```python
from build123d import *

# Parameters (mm, degrees)
SKETCH_1_R          = 1.5
EXTRUDE_2_DEPTH     = 5
CUT_EXTRUDE_2_DEPTH = 1
SKETCH_4_W          = 20
SKETCH_4_H          = 40
EXTRUDE_3_DEPTH     = 3


with BuildPart() as part:
    # 草图1 → 凸台-拉伸2 (new body)
    with BuildSketch(Plane(origin=(0, 0, 0), x_dir=(0, 0, -1), z_dir=(1, 0, 0))):
        with BuildLine():
            Line((-15, 0), (15, 0))
            Line((15, 0), (15, 130))
            ThreePointArc((15, 130), (16.060667235, 133.763397528), (17.833287426, 137.248507798))
            Line((17.833287426, 137.248507798), (34.277601095, 169.80605943))
            ThreePointArc((34.277601095, 169.80605943), (22.969406924, 178.256928012), (10.37531975, 171.878730504))
            Line((10.37531975, 171.878730504), (-12.166712574, 127.248507798))
            ThreePointArc((-12.166712574, 127.248507798), (-13.939332765, 123.763397528), (-15, 120))
            Line((-15, 120), (-15, 0))
        make_face()
        with Locations((0, 23.934052351)):
            Circle(SKETCH_1_R, mode=Mode.SUBTRACT)
        with Locations((0, 47.934052351)):
            Circle(SKETCH_1_R, mode=Mode.SUBTRACT)
        with Locations((0, 71.934052351)):
            Circle(SKETCH_1_R, mode=Mode.SUBTRACT)
        with Locations((0, 95.934052351)):
            Circle(SKETCH_1_R, mode=Mode.SUBTRACT)
        with Locations((10.541707006, 142.602806473)):
            Circle(SKETCH_1_R, mode=Mode.SUBTRACT)
        with Locations((0, 119.934052351)):
            Circle(SKETCH_1_R, mode=Mode.SUBTRACT)
        with Locations((21.812723168, 164.917917825)):
            Circle(SKETCH_1_R, mode=Mode.SUBTRACT)
        with Locations((11.964645637, 166.654399602)):
            Circle(SKETCH_1_R, mode=Mode.SUBTRACT)
        with Locations((11.964645637, 163.181436049)):
            Circle(SKETCH_1_R, mode=Mode.SUBTRACT)
        with Locations((13.15246913, 159.917917825)):
            Circle(SKETCH_1_R, mode=Mode.SUBTRACT)
        with Locations((15.384847071, 157.257473394)):
            Circle(SKETCH_1_R, mode=Mode.SUBTRACT)
        with Locations((21.812723168, 154.917917825)):
            Circle(SKETCH_1_R, mode=Mode.SUBTRACT)
        with Locations((18.392521734, 155.520991617)):
            Circle(SKETCH_1_R, mode=Mode.SUBTRACT)
        with Locations((13.15246913, 169.917917825)):
            Circle(SKETCH_1_R, mode=Mode.SUBTRACT)
        with Locations((15.384847071, 172.578362256)):
            Circle(SKETCH_1_R, mode=Mode.SUBTRACT)
        with Locations((18.392521734, 174.314844033)):
            Circle(SKETCH_1_R, mode=Mode.SUBTRACT)
        with Locations((21.812723168, 174.917917825)):
            Circle(SKETCH_1_R, mode=Mode.SUBTRACT)
    extrude(amount=-EXTRUDE_2_DEPTH)

    # 草图3 → 切除-拉伸2 (cut)
    with BuildSketch(Plane.ZY.offset(5)):
        with BuildLine():
            Line((-10, 5), (10, 5))
            Line((10, 5), (10, 119.524724411))
            ThreePointArc((10, 119.524724411), (9.161705076, 122.242477333), (7.82549521, 124.753147068))
            Line((7.82549521, 124.753147068), (-14.73885303, 169.427552317))
            ThreePointArc((-14.73885303, 169.427552317), (-21.607154469, 173.304465594), (-28.657153069, 169.768713769))
            Line((-28.657153069, 169.768713769), (-13.477541954, 139.715104809))
            ThreePointArc((-13.477541954, 139.715104809), (-11.272736422, 135.241025308), (-10, 130.418298195))
            Line((-10, 130.418298195), (-10, 5))
        make_face()
    extrude(amount=-CUT_EXTRUDE_2_DEPTH, mode=Mode.SUBTRACT)

    # 草图4 → 凸台-拉伸3 (add)
    with BuildSketch(Plane(origin=(0, 0, 0), x_dir=(-1, 0, 0), z_dir=(0, -1, 0))):
        with Locations((-5, 5)):
            Rectangle(SKETCH_4_W, SKETCH_4_H)
    extrude(amount=-EXTRUDE_3_DEPTH)


solid = part.part
```
Design review of the part built by this model. Coordinates are the model's own, in mm. A direction names the side the tool comes from. Round coordinates to 2 decimals unless told otherwise and drop trailing zeros. Write each loop counter-clockwise with the first axis right and the second up, starting at its lowest first coordinate (ties: lowest second). Pieces come first, ordered by that corner, then holes.
Item 1: For faces 1 (the flat face through (-4.51, 146.93, -17.12)), 2 (the flat face through (-2, 66, -15)), 3 (the cylindrical face through (-2.465, 175.802, -18.197)), list the 3-axis set-ups (+Z, -Z, +X, -X, +Y, -Y) from which the entire face can be reached by the end or side of a thin tool; tool diameter is ignored.
Item 2: For probe 1 along Y at (x, z) = (-1.15, 0); probe 2 along Y at (x, z) = (-3.5, -13); probe 3 along X at (y, z) = (107, 3.5), list the stretches that pass through material, from the lowest coordinate up.
Item 3: We need section D-D on z = -6.5. Write out the cut boundary in (x, y).
Item 4: Clearance check with flat-ended pins moving along their axes: pin 1 Ø4 at (y, z) = (155.52, -18.39) entering from -X; pin 2 Ø2.5 at (y, z) = (119.93, 0) entering from -X; pin 3 Ø5.5 at (x, y) = (-3.5, 47.5) entering from -Z; pin 4 Ø2 at (y, z) = (91.5, 0.5) entering from +X. State where each tip first meets the part, or that it passes through.
Item 5: The part is to be moulded in two halves that separate along Y. For faces 4 (the flat face through (-2, 55, 15)), 5 (the cylindrical face through (-4.51, 135.31, -11.3)), 6 (the cylindrical face through (-2.465, 163.247, -10.466)), 7 (the cylindrical face through (-2.465, 178.237, -23.177)), say which applies: +Y half, -Y half, draft (parallel to the pull), parting line (faces both ways), or undercut.
Item 6: We need section B-B on z = 5. Write out the cut boundary in (x, y).
Item 7: We need section A-A on y = 17.5. Write out the cut boundary in (x, z).
Item 8: We need section C-C on x = 6.5. Write out the cut boundary in (y, z), and give its area (3 significant figures).
Returned:
1. face 1: -X
1. face 2: -Z, +X, -X
1. face 3: +X, -X
2. probe 1: y = 0 to 22.43, 25.43 to 46.43, 49.43 to 70.43, 73.43 to 94.43, 97.43 to 118.43, 121.43 to 151.34
2. probe 2: y = 0 to 158.43, 161.41 to 162.1, 164.27 to 165.57, 167.74 to 168.43, 171.41 to 175
2. probe 3: x = -4 to 0
3. outline: (-5, 0) - (15, 0) - (15, 3) - (0, 3) - (0, 164.21) - (-5, 164.21) - (-5, 153.12) - (-4, 153.12) - (-4, 5) - (-5, 5) - close
4. pin 1: stops at x = -4
4. pin 2: passes through
4. pin 3: stops at z = -15
4. pin 4: stops at x = 0
5. face 4: draft
5. face 5: undercut
5. face 6: undercut
5. face 7: +Y half
6. outline: (-5, 0) - (15, 0) - (15, 3) - (0, 3) - (0, 141.44) - (-5, 141.44) - (-5, 130.35) - (-4, 130.35) - (-4, 5) - (-5, 5) - close
7. outline: (-5, -15) - (0, -15) - (0, 15) - (-5, 15) - (-5, 10) - (-4, 10) - (-4, -10) - (-5, -10) - close
8. outline: (0, -25) - (3, -25) - (3, 15) - (0, 15) - close
8. area: 120 mm2
